```python
from build123d import *

# Parameters (mm, degrees)
EXTRUDE_2_DEPTH     = 419
SKETCH_2_R          = 6
CUT_EXTRUDE_1_DEPTH = 490
SKETCH_3_R          = 15
CUT_EXTRUDE_2_DEPTH = 500


with BuildPart() as part:
    # 草图1 → 凸台-拉伸2 (new body)
    with BuildSketch(Plane.XY):
        with BuildLine():
            Line((-300, 0), (-300, -120))
            Line((-300, -120), (-303, -120))
            Line((-303, -120), (-303, 0))
            ThreePointArc((-303, 0), (0, 303), (303, 0))
            Line((303, 0), (303, -120))
            Line((303, -120), (300, -120))
            Line((300, -120), (300, 0))
            ThreePointArc((300, 0), (0, 300), (-300, 0))
        make_face()
    extrude(amount=EXTRUDE_2_DEPTH)

    # 草图2 → 切除-拉伸1 (cut)
    with BuildSketch(Plane(origin=(0, 0, 0), x_dir=(1, 0, 0), z_dir=(0, 1, 0))):
        with Locations(Location((0, -95, 0), (0, 0, 90))):
            Circle(SKETCH_2_R)
    extrude(amount=CUT_EXTRUDE_1_DEPTH, mode=Mode.SUBTRACT)

    # 草图3 → 切除-拉伸2 (cut, symmetric)
    with BuildSketch(Plane(origin=(0, 0, 0), x_dir=(0, 0, -1), z_dir=(1, 0, 0))):
        with Locations((-65, -57.08)):
            Circle(SKETCH_3_R)
    extrude(amount=CUT_EXTRUDE_2_DEPTH, both=True, mode=Mode.SUBTRACT)


solid = part.part
```
Here's how the part is built. I have some questions about the finished solid (model axes, mm). Round coordinates to 2 decimals unless told otherwise and drop trailing zeros. Order: outer loops, then holes, each group sorted by start corner. A loop starts at its lowest first (then second) coordinate and runs counter-clockwise, first axis right, second up. Notation, with made-up numbers: M 19.5,0 L 73.5,0 A16 cw 73.5,16 Z; hole C 61,7.5 d9. An arc over 180 degrees is marked long. Use CSV: the item, a comma, the result in double quotes.
1) I need wall thicknesses on line 1 along Z through (x, y) = (-301, -57); line 2 along X through (y, z) = (-17, 118); line 3 along X through (y, z) = (28, 341.5). Which ranges of each line are inside material? Lowest first, please. Write a range as [from, to].
Taken from the geometry:
line 1,"[0, 50], [80, 419]"
line 2,"[-303, -300], [300, 303]"
line 3,"[-301.7, -298.69], [298.69, 301.7]"
2) I want a section at D-D (x = 211). List the corners of the cut face in (y, z) for me, then the cut area to 3 significant figures.
Taken from the geometry:
outline,"M 213.26,0 L 217.46,0 L 217.46,419 L 213.26,419 Z"
area,"1,760 mm^2"
3) If we mould it in two halves opening along X, with no side actions, what happens to faces 1 (the flat face through (-303, -61, 207)), 2 (the flat face through (-300, -59, 207)), 3 (the cylindrical face through (301.521, -46.942, 76.056)), 4 (the flat face through (300, -61, 207))? For each: pulls with the +X half, pulls with the -X half, needs draft (parallel to the pull), parting line crosses it, or undercut.
Taken from the geometry:
face 1,"pulls with the -X half"
face 2,"undercut"
face 3,"needs draft"
face 4,"undercut"
4) I'm going to push flat-ended pins straight in: P1, Ø4, axis at x = 163.5, z = 196, coming from the +Y side; P2, Ø1, axis at y = 18.5, z = 187.5, coming from the -X side; P3, Ø4, axis at y = 123, z = 129, coming from the +X side; P4, Ø7, axis at x = 0, z = 95, coming from the -Y side. Where does each tip first touch, or does it pass through?
Taken from the geometry:
P1,"y = 256.37"
P2,"x = -302.46"
P3,"x = 277.79"
P4,"through"
5) I want a section at C-C (z = 191.5). List the corners of the cut face in (x, y) for me.
Taken from the geometry:
outline,"M -303,-120 L -300,-120 L -300,0 A300 cw 300,0 L 300,-120 L 303,-120 L 303,0 A303 ccw -303,0 Z"
6) I want a section at A-A (y = -57.08). List the corners of the cut face in (x, z) for me.
Taken from the geometry:
outline,"M -303,0 L -300,0 L -300,50 L -303,50 Z; M -303,80 L -300,80 L -300,419 L -303,419 Z; M 300,0 L 303,0 L 303,50 L 300,50 Z; M 300,80 L 303,80 L 303,419 L 300,419 Z"
7) I want a section at B-B (z = 65). List the corners of the cut face in (x, y) for me.
Taken from the geometry:
outline,"M -303,-120 L -300,-120 L -300,-72.08 L -303,-72.08 Z; M -303,-42.08 L -300,-42.08 L -300,0 A300 cw 300,0 L 300,-42.08 L 303,-42.08 L 303,0 A303 ccw -303,0 Z; M 300,-120 L 303,-120 L 303,-72.08 L 300,-72.08 Z"
